The drawing under review shows one solid part. Ordinate dimensions are in mm from its lowest x, y, z. A direction names the side the tool comes from. Give positions to 0.01 mm unless a question says otherwise; leave off trailing zeros. Write each loop counter-clockwise with the first axis right and the second up, starting at its lowest first coordinate (ties: lowest second). Pieces come first, ordered by that corner, then holes. Notation, with made-up numbers: M 50,15.25 L 89,15.25 A26 cw 89,35.25 Z; hole C 55,85 d3. An arc over 180 degrees is marked long. Write item = value, one per line. Start each with the question number.
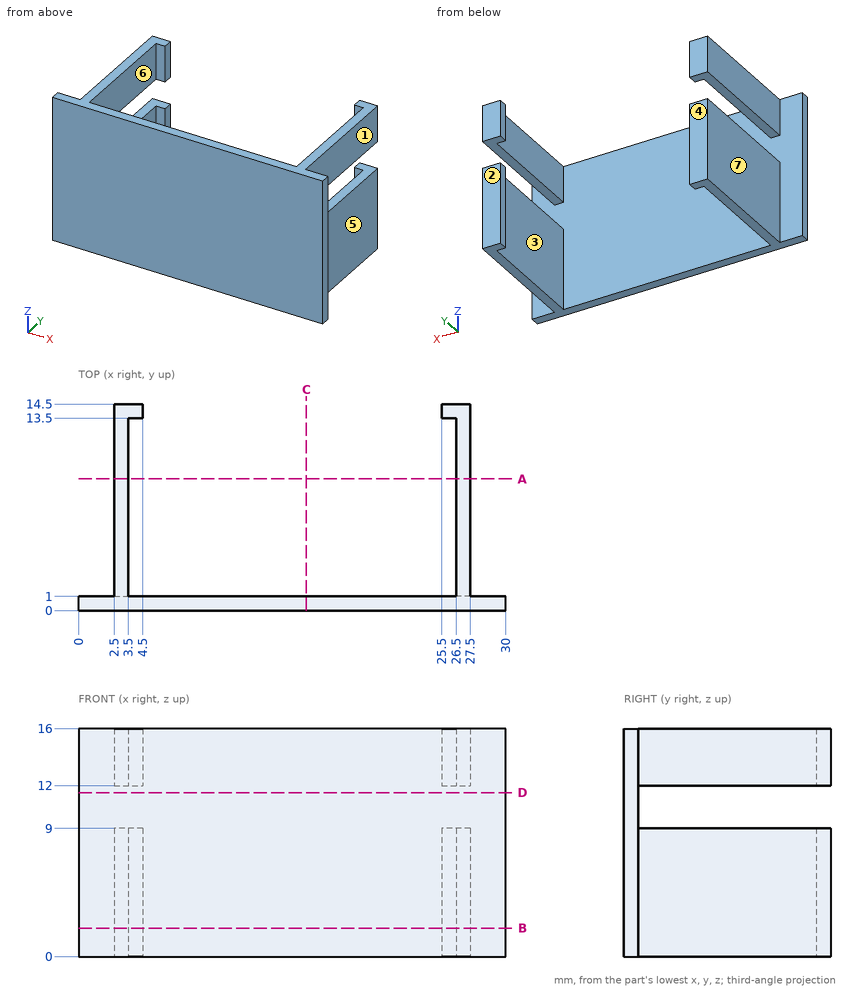
Item 1: The part is to be moulded in two halves that separate along Y. For the marked faces 1, 2 and 3, say which applies: released by +Y, released by -Y, zero draft, split by the parting line, or undercut.
Item 2: We need section B-B, the plane z = 2. Write out the cut boundary in (x, y), and give its area (3 significant figures).
Item 3: Clearance check with flat-ended pins moving along their axes: P1, Ø2.5, axis at y = 10, z = 2.5, coming from the -X side; P2, Ø1.1, axis at y = 14, z = 13, coming from the +X side; P3, Ø8, axis at x = 18.5, y = 12, coming from the +Z side. State where each tip first meets the part, or that it passes through.
Item 4: To check wall thickness, follow probe 1 along X at (y, z) = (10.25, 8.75); probe 2 along Y at (x, z) = (19.75, 5.75); probe 3 along Y at (x, z) = (26.25, 6). State the ranges of each line that lie inside material, in increasing order. Write a range as [from, to].
Item 5: We need section C-C, the plane x = 16. Write out the cut boundary in (y, z), and give its area (3 significant figures).
Item 6: We need section D-D, the plane z = 11.5. Write out the cut boundary in (x, y).
Item 7: For the marked faces 4, 5, 6 and 7, list the 3-axis set-ups (+Z, -Z, +X, -X, +Y, -Y) from which the entire face can be reached by the end or side of a thin tool; tool diameter is ignored.
Item 8: We need section A-A, the plane y = 9.25. Write out the cut boundary in (x, z), and give its area (3 significant figures).
Worked out:
q1.face_1 = zero draft
q1.face_2 = released by +Y
q1.face_3 = undercut
q2.outline = M 0,0 L 30,0 L 30,1 L 27.5,1 L 27.5,14.5 L 25.5,14.5 L 25.5,13.5 L 26.5,13.5 L 26.5,1 L 3.5,1 L 3.5,13.5 L 4.5,13.5 L 4.5,14.5 L 2.5,14.5 L 2.5,1 L 0,1 Z
q2.area = 59.0 mm²
q3.P1 = 2.5
q3.P2 = 27.5
q3.P3 = through
q4.probe_1 = [2.5, 3.5], [26.5, 27.5]
q4.probe_2 = [0, 1]
q4.probe_3 = [0, 1], [13.5, 14.5]
q5.outline = M 0,0 L 1,0 L 1,16 L 0,16 Z
q5.area = 16.0 mm²
q6.outline = M 0,0 L 30,0 L 30,1 L 0,1 Z
q7.face_4 = +Z, -Z, +X, -X, +Y
q7.face_5 = +Z, -Z, +X, +Y
q7.face_6 = +Z, -Z
q7.face_7 = +Z, -Z, -X, +Y
q8.outline = M 2.5,0 L 3.5,0 L 3.5,9 L 2.5,9 Z; M 2.5,12 L 3.5,12 L 3.5,16 L 2.5,16 Z; M 26.5,0 L 27.5,0 L 27.5,9 L 26.5,9 Z; M 26.5,12 L 27.5,12 L 27.5,16 L 26.5,16 Z
q8.area = 26.0 mm²
